Geometry: see drawing. Coordinates: mm, zero at the bounding-box minimum. Round coordinates to 2 decimals unless told otherwise and drop trailing zeros. Loops run counter-clockwise (first coordinate to the right, second up) from the corner with the lowest first, then second, coordinate; pieces in that order, holes last. Notation, with made-up numbers: (66, 22.25) - (123, 22.25) arc R35 cw to (123, 58.25) - close; hole circle Ø3 at (61.25, -23.75). An arc over 180 degrees is marked (long way). Return JSON: item names as keys, results as strings. Group by question number.
1. First-contact query: pin 1 Ø1.5 at (x, z) = (31.5, 6.5) entering from +Y. Flat tip, straight axial feed; report the tip coordinate or a pass-through.
2. Section D-D on y = 45.6. Return loops of the section in (x, z).
3. Section C-C on z = 9.5. Return loops of the section in (x, y), and give its area (3 significant figures).
4. Material intervals for probe 1 along Y at (x, z) = (18, 7.75); probe 2 along Y at (x, z) = (19, 4); probe 3 along X at (y, z) = (25.5, 6), sorted ascending.
5. Draft query along Y for the marked faces 1, 2 and 3. Return one class per face: +Y half, -Y half, draft (parallel to the pull), parting line (faces both ways), or undercut.
6. Section A-A on y = 23. Return loops of the section in (x, z), and give its area (3 significant figures).
7. Section B-B on x = 18. Return loops of the section in (y, z), and give its area (3 significant figures).
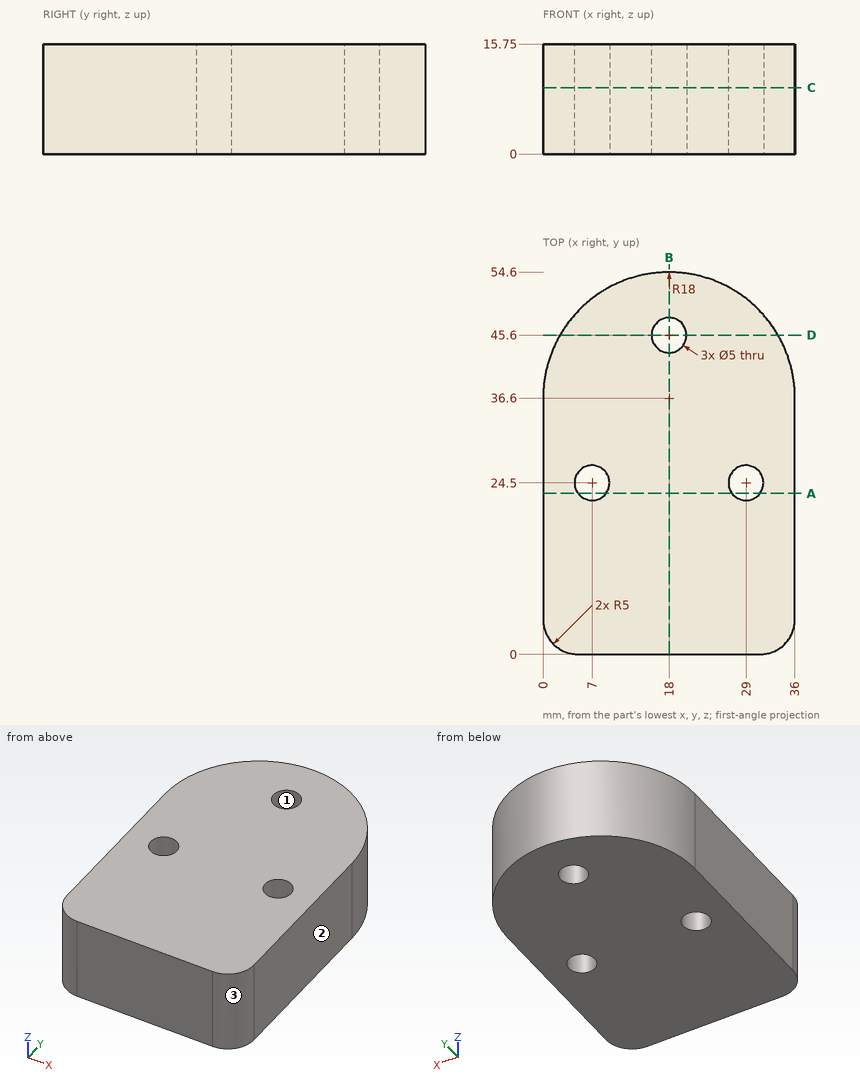
Taken from the geometry:
{
 "1": {"pin 1": "y = 49.31"},
 "2": {"outline": "(2.41, 0) - (15.5, 0) - (15.5, 15.75) - (2.41, 15.75) - close; (20.5, 0) - (33.59, 0) - (33.59, 15.75) - (20.5, 15.75) - close"},
 "3": {"outline": "(0, 5) arc R5 ccw to (5, 0) - (31, 0) arc R5 ccw to (36, 5) - (36, 36.6) arc R18 ccw to (0, 36.6) - close; hole circle Ø5 at (7, 24.5); hole circle Ø5 at (18, 45.6); hole circle Ø5 at (29, 24.5)", "area": "1,760 mm2"},
 "4": {"probe 1": "0 to 43.1, 48.1 to 54.6", "probe 2": "0 to 43.31, 47.89 to 54.57", "probe 3": "0 to 4.71, 9.29 to 26.71, 31.29 to 36"},
 "5": {"face 1": "undercut", "face 2": "draft", "face 3": "-Y half"},
 "6": {"outline": "(0, 0) - (5, 0) - (5, 15.75) - (0, 15.75) - close; (9, 0) - (27, 0) - (27, 15.75) - (9, 15.75) - close; (31, 0) - (36, 0) - (36, 15.75) - (31, 15.75) - close", "area": "441 mm2"},
 "7": {"outline": "(0, 0) - (43.1, 0) - (43.1, 15.75) - (0, 15.75) - close; (48.1, 0) - (54.6, 0) - (54.6, 15.75) - (48.1, 15.75) - close", "area": "781 mm2"}
}
